Verification items for the finished model (mm, model axes). Face numbers are marked on the shaded views. A direction names the side the tool comes from. Coordinates: 2 decimals unless noted, no trailing zeros. Order: outer loops, then holes, each group sorted by start corner. A loop starts at its lowest first (then second) coordinate and runs counter-clockwise, first axis right, second up. Notation, with made-up numbers: M 60.25,83 L 69.25,83 A31 cw 69.25,114 Z; hole C 54.25,52 d8. An arc over 180 degrees is marked long. Return JSON: item names as keys, results as strings. Group by question number.
1. Section check A-A, the plane x = 4.75. Record the cut outline in (y, z).
2. Section check C-C, the plane z = -61.5. Record the cut outline in (x, y).
3. Material ranges on line 1 along Y through (x, z) = (12.5, -28), recorded low to high.
4. Mould release check, pull along Y, two halves, no side actions. Record for the marked faces 1, 2, 3 and 4: +Y half, -Y half, draft (parallel to the pull), parting line (faces both ways), or undercut.
5. Set-up check for the marked faces 5 and 6: record each of +Z, -Z, +X, -X, +Y, -Y from which the full face is reachable in a straight line by a thin tool's end or side.
```python
from build123d import *

# Parameters (mm, degrees)
SKETCH1_W           = 25.4
SKETCH1_H           = 25.4
SKETCH1_W_2         = 22.9108
SKETCH1_H_2         = 22.9108
BOSS_EXTRUDE1_DEPTH = 152.4
FILLET1_R           = 0.4064
FILLET2_R           = 0.4064
SKETCH2_R           = 3.96875
CUT_EXTRUDE1_DEPTH  = 157.576115675


with BuildPart() as part:
    # Sketch1 → Boss-Extrude1 (new body)
    with BuildSketch(Plane.XY):
        with Locations((12.7, 12.7)):
            Rectangle(SKETCH1_W, SKETCH1_H)
        with Locations((12.7, 12.7)):
            Rectangle(SKETCH1_W_2, SKETCH1_H_2, mode=Mode.SUBTRACT)
    extrude(amount=-BOSS_EXTRUDE1_DEPTH)

    # Fillet1
    fillet1_edges = [part.edges().sort_by_distance(p)[0] for p in [
        (0, 25.4, -76.2),
        (25.4, 25.4, -76.2),
        (25.4, 0, -76.2),
        (0, 0, -76.2),
    ]]
    fillet(fillet1_edges, radius=FILLET1_R)

    # Fillet2
    fillet2_edges = [part.edges().sort_by_distance(p)[0] for p in [
        (1.2446, 1.2446, -76.2),
        (1.2446, 24.1554, -76.2),
        (24.1554, 24.1554, -76.2),
        (24.1554, 1.2446, -76.2),
    ]]
    fillet(fillet2_edges, radius=FILLET2_R)

    # Sketch2 → Cut-Extrude1 (cut, through all)
    with BuildSketch(Plane(origin=(0, 25.4, 0), x_dir=(1, 0, 0), z_dir=(0, 1, 0))):
        with Locations((12.7, 0)):
            Circle(SKETCH2_R)
    extrude(amount=-CUT_EXTRUDE1_DEPTH, mode=Mode.SUBTRACT)


solid = part.part
```
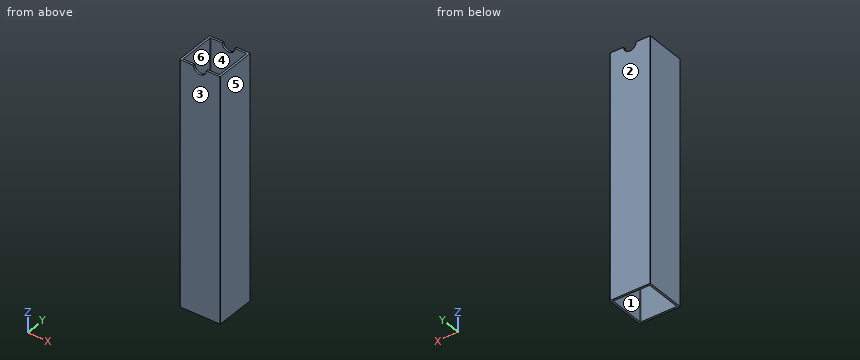
Answers follow:
{
 "1": {"outline": "M 0,-152.4 L 1.24,-152.4 L 1.24,0 L 0,0 Z; M 24.16,-152.4 L 25.4,-152.4 L 25.4,0 L 24.16,0 Z"},
 "2": {"outline": "M 0,0.41 A0.41 ccw 0.41,0 L 24.99,0 A0.41 ccw 25.4,0.41 L 25.4,24.99 A0.41 ccw 24.99,25.4 L 0.41,25.4 A0.41 ccw 0,24.99 Z; hole M 1.24,1.65 A0.41 ccw 1.65,1.24 L 23.75,1.24 A0.41 ccw 24.16,1.65 L 24.16,23.75 A0.41 ccw 23.75,24.16 L 1.65,24.16 A0.41 ccw 1.24,23.75 Z"},
 "3": {"line 1": "0 to 1.24, 24.16 to 25.4"},
 "4": {"face 1": "undercut", "face 2": "+Y half", "face 3": "-Y half", "face 4": "undercut"},
 "5": {"face 5": "+Z, -Z, +X, +Y, -Y", "face 6": "+Z, -Z"}
}
